Design review of the part shown in the three views and the two pictorial views. Dimensions are in mm from the part's minimum x, y and z. A direction names the side the tool comes from. Round coordinates to 2 decimals unless told otherwise and drop trailing zeros. Order: outer loops, then holes, each group sorted by start corner. A loop starts at its lowest first (then second) coordinate and runs counter-clockwise, first axis right, second up. Notation, with made-up numbers: M -29.75,47 L 4.25,47 A19 cw 4.25,67 Z; hole C 35,39 d7. An arc over 180 degrees is marked long. Write item = value, one per line. Start each with the question number.
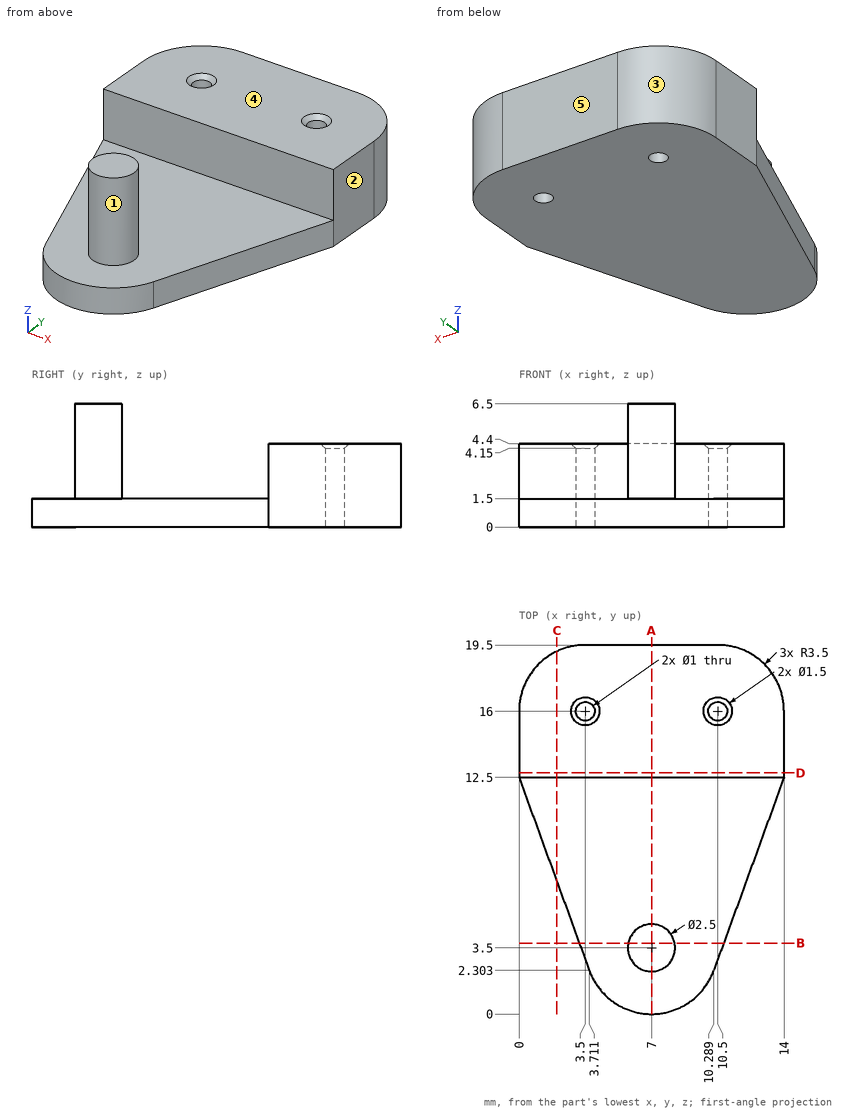
(1) We need section A-A, the plane x = 7. Write out the cut boundary in (y, z).
(2) We need section C-C, the plane x = 2. Write out the cut boundary in (y, z).
(3) Draft analysis for pull direction Y (two halves, no side actions). For the marked faces 1, 2 and 3, state which applies: released by +Y, released by -Y, zero draft, split by the parting line, or undercut.
(4) For the marked faces 4 and 5, list the 3-axis set-ups (+Z, -Z, +X, -X, +Y, -Y) from which the entire face can be reached by the end or side of a thin tool; tool diameter is ignored.
(5) We need section B-B, the plane y = 3.75. Write out the cut boundary in (x, z).
(6) We need section D-D, the plane y = 12.75. Write out the cut boundary in (x, z).
(7) Insertion check: pin 1 (1 mm diameter, centred on x = 5, y = 4, fed in from +Z); pin 2 (2 mm diameter, centred on x = 5.5, y = 15, fed in from +Z); pin 3 (6.5 mm diameter, centred on x = 9.5, y = 5, fed in from +Z); pin 4 (2.5 mm diameter, centred on x = 8.5, z = 2.5, fed in from -Y). Each pin has a flat end and moves straight along its axis. Give the tip position at first contact, or say it passes through.
(8) For line 1 along Y through (x, z) = (3.5, 2.1); line 2 along Z through (x, y) = (4.75, 2.25); line 3 along Z through (x, y) = (9.25, 14.5), list the stretches that pass through material, from the lowest coordinate up.
Values:
q1.outline = M 0,0 L 19.5,0 L 19.5,4.4 L 12.5,4.4 L 12.5,1.5 L 4.75,1.5 L 4.75,6.5 L 2.25,6.5 L 2.25,1.5 L 0,1.5 Z
q2.outline = M 7,0 L 19.16,0 L 19.16,4.4 L 12.5,4.4 L 12.5,1.5 L 7,1.5 Z
q3.face_1 = undercut
q3.face_2 = zero draft
q3.face_3 = released by +Y
q4.face_4 = +Z, +X, -X, +Y
q4.face_5 = +Z, -Z, +X, -X, +Y
q5.outline = M 3.18,0 L 10.82,0 L 10.82,1.5 L 8.22,1.5 L 8.22,6.5 L 5.78,6.5 L 5.78,1.5 L 3.18,1.5 Z
q6.outline = M 0,0 L 14,0 L 14,4.4 L 0,4.4 Z
q7.pin_1 = 1.5
q7.pin_2 = 4.4
q7.pin_3 = 6.5
q7.pin_4 = 0.08
q8.line_1 = 12.5 to 15.5, 16.5 to 19.5
q8.line_2 = 0 to 1.5
q8.line_3 = 0 to 4.4
